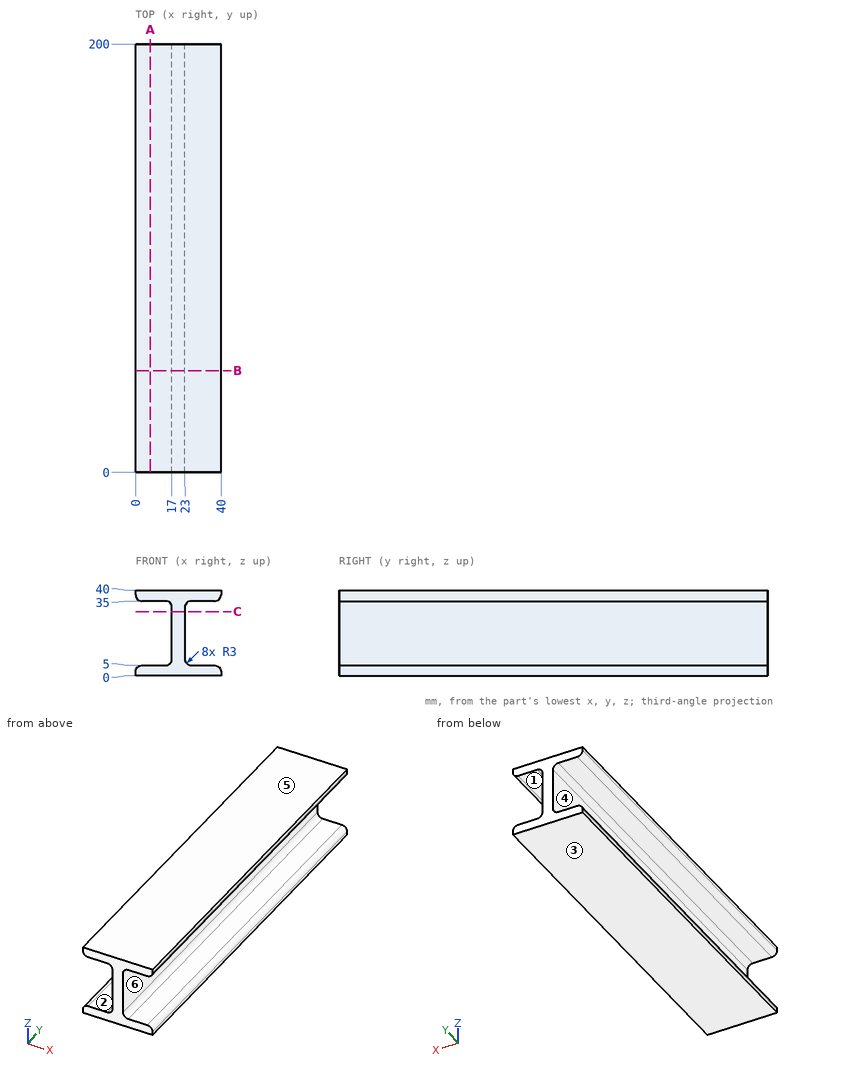
Here's the drawing with two shaded views (mm, measured from the low corner). I have some questions. A direction names the side the tool comes from. Give positions to 0.01 mm unless a question says otherwise; leave off trailing zeros. Order: outer loops, then holes, each group sorted by start corner. A loop starts at its lowest first (then second) coordinate and runs counter-clockwise, first axis right, second up. Notation, with made-up numbers: (26, 73) -> (46, 73) arc R22 cw to (46, 106) -> close; hole circle Ø1 at (56.25, -0.75). An arc over 180 degrees is marked (long way). Use a Markdown table: item, result. Add a question column.
Item 1: If we mould it in two halves opening along Z, with no side actions, what happens to the marked faces 3, 4, 5 and 6? For each: pulls with the +Z half, pulls with the -Z half, needs draft (parallel to the pull), parting line crosses it, or undercut.
Item 2: For the marked faces 1 and 2, which set-ups out of +Z, -Z, +X, -X, +Y, -Y let a thin tool reach every point of the face, with its end or its side?
Item 3: Imagine slicing it at B-B on y = 47.5. Please give me the cut outline in (x, z).
Item 4: Imagine slicing it at C-C on z = 30. Please give me the cut outline in (x, y), plus the area to 3 significant figures.
Item 5: Will these pins go through, and if not, where does the flat tip stop? pin 1 (19 mm diameter, centred on y = 120.5, z = 17.5, fed in from -X); pin 2 (19 mm diameter, centred on y = 145, z = 18.5, fed in from +X); pin 3 (3 mm diameter, centred on y = 175.5, z = 8, fed in from +X).
Item 6: I need wall thicknesses on line 1 (Z direction, x = 37, y = 78); line 2 (X direction, y = 87.5, z = 29.5); line 3 (Z direction, x = 16, y = 139). Which ranges of each line are inside material? Lowest first, please.
Item 7: Imagine slicing it at A-A on x = 7. Please give me the cut outline in (y, z).
Data:
| question | item | result |
|---|---|---|
| 1 | face 3 | pulls with the -Z half |
| 1 | face 4 | undercut |
| 1 | face 5 | pulls with the +Z half |
| 1 | face 6 | undercut |
| 2 | face 1 | +X, +Y, -Y |
| 2 | face 2 | -X, +Y, -Y |
| 3 | outline | (0, 0) -> (40, 0) -> (40, 2) arc R3 ccw to (37, 5) -> (26, 5) arc R3 cw to (23, 8) -> (23, 32) arc R3 cw to (26, 35) -> (37, 35) arc R3 ccw to (40, 38) -> (40, 40) -> (0, 40) -> (0, 38) arc R3 ccw to (3, 35) -> (14, 35) arc R3 cw to (17, 32) -> (17, 8) arc R3 cw to (14, 5) -> (3, 5) arc R3 ccw to (0, 2) -> close |
| 4 | outline | (17, 0) -> (23, 0) -> (23, 200) -> (17, 200) -> close |
| 4 | area | 1,200 mm² |
| 5 | pin 1 | stops at x = 17 |
| 5 | pin 2 | stops at x = 23 |
| 5 | pin 3 | stops at x = 23.4 |
| 6 | line 1 | z = 0 to 5, 35 to 40 |
| 6 | line 2 | x = 17 to 23 |
| 6 | line 3 | z = 0 to 5.76, 34.24 to 40 |
| 7 | outline | (0, 0) -> (200, 0) -> (200, 5) -> (0, 5) -> close; (0, 35) -> (200, 35) -> (200, 40) -> (0, 40) -> close |
